The model under review builds one solid part; all positions refer to its coordinate system, in mm. Face numbers are marked on the shaded views. A direction names the side the tool comes from. Coordinates: 2 decimals unless noted, no trailing zeros. Write each loop counter-clockwise with the first axis right and the second up, starting at its lowest first coordinate (ties: lowest second). Pieces come first, ordered by that corner, then holes. Notation, with made-up numbers: M 8.5,79.5 L 18.5,79.5 A22 cw 18.5,117.5 Z; hole C 21,42.25 d5. An arc over 180 degrees is marked long. Answer as a JSON object with one key per item and string values.
```python
from build123d import *

# Parameters (mm, degrees)
BASPROSKE_W           = 3
BASPROSKE_H           = 14.25
TOOTHCUT_DEPTH        = 21.374616561
TEETHCUTS_COUNT       = 17
TEETHCUTS_ANGLE       = 338.823529412
BORSKE_R              = 2.5
BORE_DEPTH            = 50.0000508
CROQUIS1_R            = 1.5
CROQUIS1_R_2          = 3.625
CORTAR_EXTRUIR1_DEPTH = 10


with BuildPart() as part:
    # BasProSke → Base-Revolve (revolve)
    with BuildSketch(Plane(origin=(0, 0, 0), x_dir=(1, 0, 0), z_dir=(0, 1, 0)), mode=Mode.PRIVATE) as base_revolve_sk:
        with Locations((1.5, 7.125)):
            Rectangle(BASPROSKE_W, BASPROSKE_H)
    revolve(base_revolve_sk.sketch.rotate(Axis((-10, 0, 0), (1, 0, 0)), 180), axis=Axis((-10, 0, 0), (1, 0, 0)))

    # TooCutSke → ToothCut (cut, through all)
    with BuildSketch(Plane(origin=(0, 0, 0), x_dir=(0, 0, -1), z_dir=(1, 0, 0))):
        with BuildLine():
            ThreePointArc((0.769354207, 10.846749287), (0, 10.874), (-0.769354207, 10.846749287))
            ThreePointArc((-0.769354207, 10.846749287), (-1.230849554, 12.606357238), (-2.280560064, 14.092057726))
            ThreePointArc((-2.280560064, 14.092057726), (0, 14.2754), (2.280560064, 14.092057726))
            ThreePointArc((2.280560064, 14.092057726), (1.230849554, 12.606357238), (0.769354207, 10.846749287))
        make_face()
    toothcut = extrude(amount=TOOTHCUT_DEPTH, mode=Mode.SUBTRACT)

    # TeethCuts: ToothCut ×17 about axis
    teethcuts_axis = Axis((-10, 0, 0), (1, 0, 0))
    for i in range(1, TEETHCUTS_COUNT):
        add(toothcut.rotate(teethcuts_axis, i * TEETHCUTS_ANGLE / (TEETHCUTS_COUNT - 1)), mode=Mode.SUBTRACT)

    # BorSke → Bore (cut, symmetric)
    with BuildSketch(Plane(origin=(0, 0, 0), x_dir=(0, 0, -1), z_dir=(1, 0, 0))):
        with Locations(Location((0, 0, 0), (0, 0, 180))):
            Circle(BORSKE_R)
    extrude(amount=BORE_DEPTH, both=True, mode=Mode.SUBTRACT)

    # Croquis1 → Cortar-Extruir1 (cut)
    with BuildSketch(Plane(origin=(3, 0, 0), x_dir=(0, 0, -1), z_dir=(1, 0, 0))):
        with Locations((7.25, 0)):
            Circle(CROQUIS1_R)
        Circle(CROQUIS1_R_2)
        with Locations((-7.25, 0)):
            Circle(CROQUIS1_R)
    extrude(amount=-CORTAR_EXTRUIR1_DEPTH, mode=Mode.SUBTRACT)


solid = part.part
```
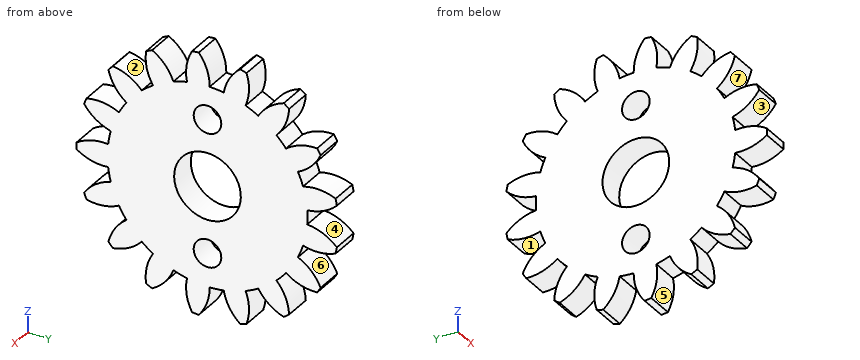
(1) Wall thickness on line 1 along Y through (x, z) = (0.25, -12.25); line 2 along Y through (x, z) = (0.1, -8.5); line 3 along Y through (x, z) = (1.8, 0) (3 decimals): over which ranges is each line inside the solid? List them lowest first. Write a range as from..to.
Results list:
{"line 1": "-6.71..-5.09, -2.3..0.07, 2.28..4.51", "line 2": "-10.51..-7.45, -6.78..-0.83, 0.83..8", "line 3": "-14.25..-3.625, 3.625..10.874"}
(2) Add section B-B on y = 3. Give the boundary of the cut face in (x, z), and give its area (3 significant figures).
Results list:
{"outline": "M 0,-13.28 L 3,-13.28 L 3,-2.03 L 0,-2.03 Z; M 0,2.03 L 3,2.03 L 3,13.28 L 0,13.28 Z", "area": "67.5 mm²"}
(3) Add section D-D on x = 0.9. Count the separate pieces of the cut face and the enclosed holes in it, and give its area (3 significant figures).
Results list:
{"separate pieces": "1", "enclosed holes": "3", "area": "434 mm²"}
(4) Add section A-A on z = 0. Give the boundary of the cut face in (x, y) (3 decimals).
Results list:
{"outline": "M 0,-14.25 L 3,-14.25 L 3,-3.625 L 0,-3.625 Z; M 0,3.625 L 3,3.625 L 3,10.874 L 0,10.874 Z"}
(5) Add section C-C on z = 12. Give the boundary of the cut face in (x, y).
Results list:
{"outline": "M 0,-6.73 L 3,-6.73 L 3,-4.83 L 0,-4.83 Z; M 0,-2.32 L 3,-2.32 L 3,0.13 L 0,0.13 Z; M 0,2.16 L 3,2.16 L 3,4.52 L 0,4.52 Z"}
(6) Draft analysis for pull direction Y (two halves, no side actions). For the marked faces 5, 6 and 7, state which applies: released by +Y, released by -Y, zero draft, split by the parting line, or undercut.
Results list:
{"face 5": "undercut", "face 6": "released by +Y", "face 7": "released by -Y"}
(7) For pin 1 Ø1.5 at (y, z) = (-1.5, -2) entering from +X, flat-tipped, find the tip position at first contact; note if it passes through.
Results list:
{"pin 1": "through"}
(8) For the marked faces 1, 2, 3 and 4, list the 3-axis set-ups (+Z, -Z, +X, -X, +Y, -Y) from which the entire face can be reached by the end or side of a thin tool; tool diameter is ignored.
Results list:
{"face 1": "+X, -X", "face 2": "+Z, +X, -X", "face 3": "+X, -X, -Y", "face 4": "+X, -X, +Y"}
